Geometry: see drawing. Coordinates: mm, zero at the bounding-box minimum. A direction names the side the tool comes from. Give positions to 0.01 mm unless a question says otherwise; leave off trailing zeros. Write each loop counter-clockwise with the first axis right and the second up, starting at its lowest first coordinate (ties: lowest second). Pieces come first, ordered by that corner, then holes. Notation, with made-up numbers: (82, 33) -> (128, 33) arc R11 ccw to (128, 43) -> close; hole circle Ø3 at (-29.75, 32). An arc over 180 degrees is marked (long way). Use one line per item in the form item = value. Start each with the question number.
(1) Cut plane B-B, the plane z = 4.75. Count the separate pieces of the cut face and the enclosed holes in it, and give its area (3 significant figures).
(2) Cut plane D-D, the plane x = 100. Output: boundary loops of the cut face in (y, z) (3 decimals), and give its area (3 significant figures).
(3) Set-up query: the marked faces 1, 2 and 3. Return all of +Z, -Z, +X, -X, +Y, -Y with unobstructed straight access to the full face (end or side cutting, diameter ignored); none if empty.
(4) Cut plane A-A, the plane x = 50. Output: boundary loops of the cut face in (y, z) (3 decimals), and give its area (3 significant figures).
(5) Cut plane C-C, the plane x = 205. Output: boundary loops of the cut face in (y, z) (3 decimals), and give its area (3 significant figures).
(6) Material intervals for line 1 along Y through (x, z) = (205, 5.25); line 2 along Y through (x, z) = (160, 6.5); line 3 along Y through (x, z) = (48, 6), sorted ascending. Write a range as from..to.
(7) Draft query along X for the marked faces 4, 5 and 6. Return one class per face: pulls with the +X half, pulls with the -X half, needs draft (parallel to the pull), parting line crosses it, or undercut.
(8) First-contact query: P1, Ø8, axis at x = 7, z = 5.5, coming from the -Y side; P2, Ø1, axis at x = 135, z = 3.5, coming from the -Y side; P3, Ø5, axis at x = 130, y = 30, coming from the +Z side. Flat tips, straight axial feed; report the tip coordinate or a pass-through.
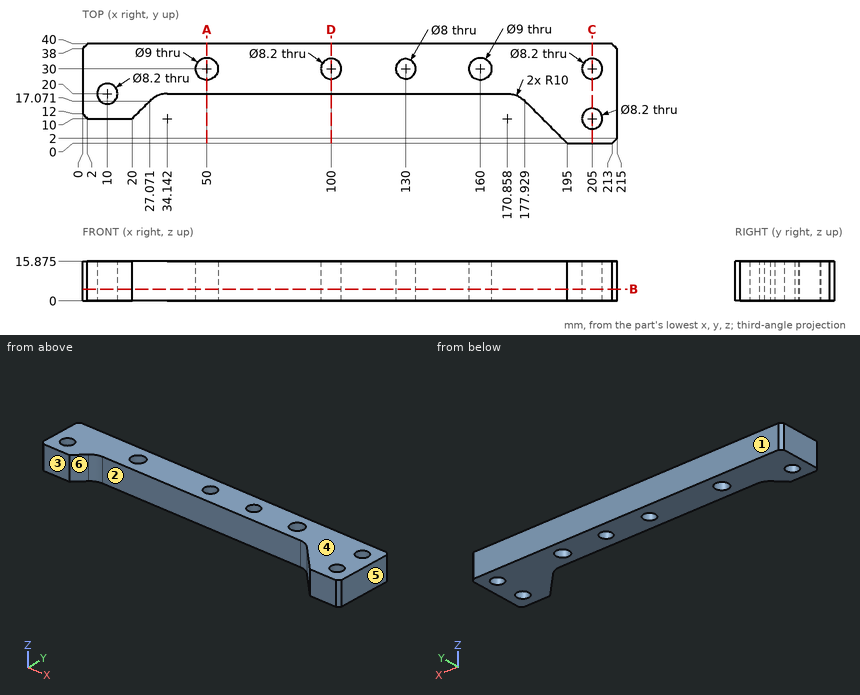
Geometry says:
q1.separate_pieces = 1
q1.enclosed_holes = 7
q1.area = 4,760 mm^2
q2.outline = (20, 0) -> (25.9, 0) -> (25.9, 15.875) -> (20, 15.875) -> close; (34.1, 0) -> (40, 0) -> (40, 15.875) -> (34.1, 15.875) -> close
q2.area = 187 mm^2
q3.face_1 = +Z, -Z, +X, -X, +Y
q3.face_2 = +Z, -Z, -Y
q3.face_3 = +Z, -Z, -X, -Y
q4.outline = (20, 0) -> (25.5, 0) -> (25.5, 15.875) -> (20, 15.875) -> close; (34.5, 0) -> (40, 0) -> (40, 15.875) -> (34.5, 15.875) -> close
q4.area = 175 mm^2
q5.outline = (0, 0) -> (5.9, 0) -> (5.9, 15.875) -> (0, 15.875) -> close; (14.1, 0) -> (25.9, 0) -> (25.9, 15.875) -> (14.1, 15.875) -> close; (34.1, 0) -> (40, 0) -> (40, 15.875) -> (34.1, 15.875) -> close
q5.area = 375 mm^2
q6.line_1 = 0..5.9, 14.1..25.9, 34.1..40
q6.line_2 = 20..25.5, 34.5..40
q6.line_3 = 20..25.97, 34.03..40
q7.face_4 = needs draft
q7.face_5 = pulls with the +X half
q7.face_6 = undercut
q8.P1 = 10
q8.P2 = 20
q8.P3 = through
